Geometry check sheet. Reference: the model listing, model coordinates, mm. A direction names the side the tool comes from. Coordinates: 2 decimals unless noted, no trailing zeros. Write each loop counter-clockwise with the first axis right and the second up, starting at its lowest first coordinate (ties: lowest second). Pieces come first, ordered by that corner, then holes.
from build123d import *

# Parameters (mm, degrees)
ESQUISSE1_W             = 20
ESQUISSE1_H             = 17
BOSS_EXTRU_1_DEPTH      = 6
ESQUISSE2_R             = 15.5
BOSS_EXTRU_2_DEPTH      = 6
ESQUISSE3_R             = 12.55
ENL_V_MAT_EXTRU_1_DEPTH = 6
ESQUISSE4_W             = 10
ESQUISSE4_H             = 11.989026974
ENL_V_MAT_EXTRU_2_DEPTH = 10


with BuildPart() as part:
    # Esquisse1 → Boss.-Extru.1 (new body)
    with BuildSketch(Plane.XY):
        Rectangle(ESQUISSE1_W, ESQUISSE1_H)
    extrude(amount=BOSS_EXTRU_1_DEPTH)

    # Esquisse2 → Boss.-Extru.2 (add)
    with BuildSketch(Plane.XY.offset(6)):
        with Locations((0, 18)):
            Circle(ESQUISSE2_R)
    extrude(amount=-BOSS_EXTRU_2_DEPTH)

    # Esquisse3 → Enlèv. mat.-Extru.1 (cut)
    with BuildSketch(Plane.XY.offset(6)):
        with Locations((0, 18)):
            Circle(ESQUISSE3_R)
    extrude(amount=-ENL_V_MAT_EXTRU_1_DEPTH, mode=Mode.SUBTRACT)

    # Esquisse4 → Enlèv. mat.-Extru.2 (cut)
    with BuildSketch(Plane.XY.offset(6)):
        with Locations((0, 0.494513487)):
            Rectangle(ESQUISSE4_W, ESQUISSE4_H)
    extrude(amount=-ENL_V_MAT_EXTRU_2_DEPTH, mode=Mode.SUBTRACT)


solid = part.part
1. Sectioned sample at D-D, the plane x = 13. Record the boundary of the cut face in (y, z), and give its area (3 significant figures).
Computed values:
outline: (9.56, 0) - (26.44, 0) - (26.44, 6) - (9.56, 6) - close
area: 101 mm2
2. Gauge pin test, flat ends, axial feed: pin 1 Ø1.5 at (y, z) = (8, 2.5) entering from +X; pin 2 Ø1.8 at (y, z) = (-2.5, 4) entering from +X; pin 3 Ø8 at (x, y) = (-6.5, 22.5) entering from -Z; pin 4 Ø3 at (y, z) = (-4, 3) entering from -X. Record the tip position at first contact, or that the pin passes through.
Computed values:
pin 1: stops at x = 12.44
pin 2: stops at x = 10
pin 3: passes through
pin 4: stops at x = -10
3. Sectioned sample at B-B, the plane z = 3.2. Record the boundary of the cut face in (x, y).
Computed values:
outline: (-10, -8.5) - (10, -8.5) - (10, 6.16) arc R15.5 ccw (long way) to (-10, 6.16) - close; hole (-5, -5.5) - (5, -5.5) - (5, 6.49) arc R12.55 ccw (long way) to (-5, 6.49) - close
4. Sectioned sample at A-A, the plane x = 0. Record the boundary of the cut face in (y, z), and give its area (3 significant figures).
Computed values:
outline: (-8.5, 0) - (-5.5, 0) - (-5.5, 6) - (-8.5, 6) - close; (30.55, 0) - (33.5, 0) - (33.5, 6) - (30.55, 6) - close
area: 35.7 mm2
5. Sectioned sample at C-C, the plane y = 18. Record the boundary of the cut face in (x, z), and give its area (3 significant figures).
Computed values:
outline: (-15.5, 0) - (-12.55, 0) - (-12.55, 6) - (-15.5, 6) - close; (12.55, 0) - (15.5, 0) - (15.5, 6) - (12.55, 6) - close
area: 35.4 mm2
6. Access from +Z, -Z, +X, -X, +Y, -Y to the whole of each face (thin tool, end or side, straight path). Record for faces 1 (the flat face through (10, -1, 3)), 2 (the flat face through (-5, 0, 3)), 3 (the flat face through (0, -8.5, 3)).
Computed values:
face 1: +Z, -Z, +X, -Y
face 2: +Z, -Z
face 3: +Z, -Z, +X, -X, -Y
7. Thickness scan on line 1 along Y through (x, z) = (0, 2.55); line 2 along X through (y, z) = (5.5, 3.7); line 3 along X through (y, z) = (18, 1.5). Record the ranges inside material, lowest first.
Computed values:
line 1: y = -8.5 to -5.5, 30.55 to 33.5
line 2: x = -10 to -5, 5 to 10
line 3: x = -15.5 to -12.55, 12.55 to 15.5
8. Draft check along X on faces 4 (the flat face through (5, 0, 3)), 5 (the flat face through (0, -5.5, 3)), 6 (the flat face through (-6, 6, 0)), 7 (the flat face through (-10, -1, 3)). Enter one of: released by +X, released by -X, zero draft, split by the parting line, or undercut.
Computed values:
face 4: undercut
face 5: undercut
face 6: zero draft
face 7: released by -X
